Answer from the drawing. Dimensions are ordinates in mm from the lowest x, y and z of the part. Give positions to 0.01 mm unless a question says otherwise; leave off trailing zeros. Loops run counter-clockwise (first coordinate to the right, second up) from the corner with the lowest first, then second, coordinate; pieces in that order, holes last.
(1) Find section B-B, the plane y = 5.25. Write down the section's boundary in (x, z) (3 decimals).
(2) Find section A-A, the plane z = 1.35. Write down the section's boundary in (x, y) (3 decimals), then the cut area to 3 significant figures.
(3) Straight lines are drawn through the part: probe 1 along X at (y, z) = (5.5, 1.6); probe 2 along X at (y, z) = (2.5, 0.45). For each, find the intervals that lie inside material, in ascending order.
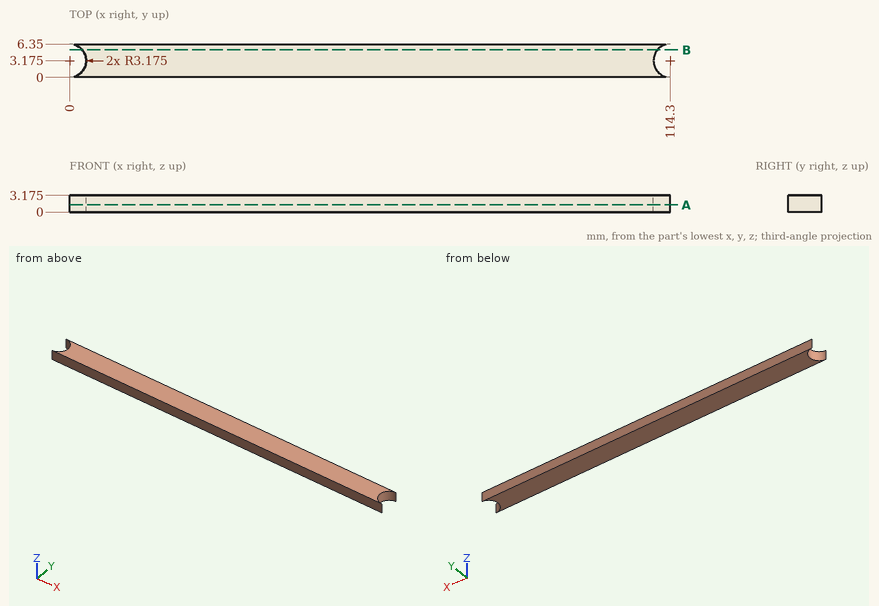
Entries:
1. outline: (2.403, 0) - (111.897, 0) - (111.897, 3.175) - (2.403, 3.175) - close
2. outline: (0, 0) - (114.3, 0) arc R3.175 cw to (114.3, 6.35) - (0, 6.35) arc R3.175 cw to start
2. area: 694 mm2
3. probe 1: x = 2.16 to 112.14
3. probe 2: x = 3.1 to 111.2
